Print and shaded views of the part. All mm, measured from the part's lowest x, y and z. Round coordinates to 2 decimals unless told otherwise and drop trailing zeros. Loops run counter-clockwise (first coordinate to the right, second up) from the corner with the lowest first, then second, coordinate; pieces in that order, holes last. Notation, with made-up numbers: (77, 21.25) - (99, 21.25) arc R26 ccw to (99, 56.25) - close; hole circle Ø10 at (-20, 16.5). An arc over 180 degrees is marked (long way). Use one line per item in the form item = value.
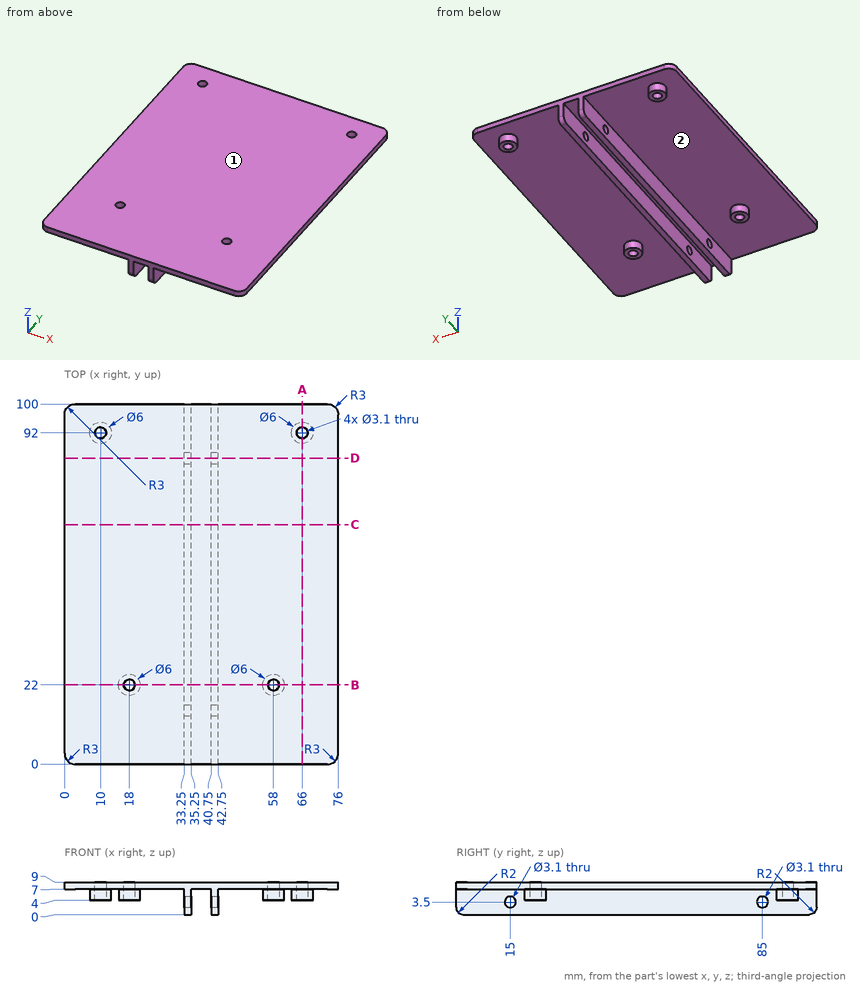
1) Two-plate mould, pull along Z, no slides. Class the marked faces 1 and 2: +Z half, -Z half, draft (parallel to the pull), parting line (faces both ways), or undercut.
Report:
face_1 = +Z half
face_2 = -Z half
2) Drill centre lines: probe 1 along Y at (x, z) = (41.65, 3.5); probe 2 along X at (y, z) = (29, 1.5); probe 3 along Y at (x, z) = (66, 6). Where is each one in solid material? Low to high.
Report:
probe_1 = 0 to 13.45, 16.55 to 83.45, 86.55 to 100
probe_2 = 33.25 to 35.25, 40.75 to 42.75
probe_3 = 89 to 90.45, 93.55 to 95
3) Slice it at B-B (y = 22). Write the cut outline in (x, z).
Report:
outline = (0, 7) - (15, 7) - (15, 4) - (16.45, 4) - (16.45, 9) - (0, 9) - close; (19.55, 4) - (21, 4) - (21, 7) - (33.25, 7) - (33.25, 0) - (35.25, 0) - (35.25, 7) - (40.75, 7) - (40.75, 0) - (42.75, 0) - (42.75, 7) - (55, 7) - (55, 4) - (56.45, 4) - (56.45, 9) - (19.55, 9) - close; (59.55, 4) - (61, 4) - (61, 7) - (76, 7) - (76, 9) - (59.55, 9) - close
4) Slice it at C-C (y = 66.5). Write the cut outline in (x, z).
Report:
outline = (0, 7) - (33.25, 7) - (33.25, 0) - (35.25, 0) - (35.25, 7) - (40.75, 7) - (40.75, 0) - (42.75, 0) - (42.75, 7) - (76, 7) - (76, 9) - (0, 9) - close
5) Slice it at D-D (y = 85). Write the cut outline in (x, z).
Report:
outline = (0, 7) - (33.25, 7) - (33.25, 5.05) - (35.25, 5.05) - (35.25, 7) - (40.75, 7) - (40.75, 5.05) - (42.75, 5.05) - (42.75, 7) - (76, 7) - (76, 9) - (0, 9) - close; (33.25, 0) - (35.25, 0) - (35.25, 1.95) - (33.25, 1.95) - close; (40.75, 0) - (42.75, 0) - (42.75, 1.95) - (40.75, 1.95) - close
6) Slice it at A-A (x = 66). Write the cut outline in (y, z), plus the area to 4 significant figures.
Report:
outline = (0, 7) - (89, 7) - (89, 4) - (90.45, 4) - (90.45, 9) - (0, 9) - close; (93.55, 4) - (95, 4) - (95, 7) - (100, 7) - (100, 9) - (93.55, 9) - close
area = 202.5 mm^2
7) Flat gauge pins, fed straight in: pin 1 (5 mm diameter, centred on y = 85, z = 3.5, fed in from -X); pin 2 (6.5 mm diameter, centred on x = 66.5, y = 91, fed in from -Z); pin 3 (2 mm diameter, centred on y = 64, z = 5, fed in from +X). Where does each tip first touch, or does it go through?
Report:
pin_1 = 33.25
pin_2 = 4
pin_3 = 42.75
